Geometry: final body of the model. Coordinates: model frame, mm. Face numbers are marked on the shaded views. Round coordinates to 2 decimals unless told otherwise and drop trailing zeros. Loops run counter-clockwise (first coordinate to the right, second up) from the corner with the lowest first, then second, coordinate; pieces in that order, holes last. Notation, with made-up numbers: (2, 51) - (8, 51) arc R21 cw to (8, 66) - close; hole circle Ø6 at (43, -17). An arc over 180 degrees is marked (long way). Answer as a JSON object with one key per item and string values. Group by question number.
Item 1: Section B-B (y = 0). Return the cut outline in (x, z).
Item 2: Line query: line 1 (Y direction, x = 12, z = 0); line 2 (Z direction, x = 11.75, y = 3); line 3 (Y direction, x = 14, z = 6.5). Output: solid intervals per line, ascending.
Item 3: Section A-A (z = 0). Return the cut outline in (x, y), plus the area to 3 significant figures.
Item 4: Draft query along Y for the marked faces 1, 2 and 3. Return one class per face: released by +Y, released by -Y, zero draft, split by the parting line, or undercut.
Item 5: Section C-C (x = 6). Return the cut outline in (y, z).
```python
from build123d import *

# Parameters (mm, degrees)
SKETCH1_W           = 35
SKETCH1_H           = 30
BOSS_EXTRUDE1_DEPTH = 25
SKETCH2_R           = 8.23
CUT_EXTRUDE1_DEPTH  = 51
SKETCH3_W           = 35
SKETCH3_H           = 30
CUT_EXTRUDE2_DEPTH  = 5
SKETCH4_W           = 35
SKETCH4_H           = 30
CUT_EXTRUDE3_DEPTH  = 5


with BuildPart() as part:
    # Sketch1 → Boss-Extrude1 (new body)
    with BuildSketch(Plane(origin=(0, 0, 0), x_dir=(0, 0, -1), z_dir=(1, 0, 0))):
        Rectangle(SKETCH1_W, SKETCH1_H)
    extrude(amount=BOSS_EXTRUDE1_DEPTH)

    # Sketch2 → Cut-Extrude1 (cut)
    with BuildSketch(Plane(origin=(25, 0, 0), x_dir=(0, 0, -1), z_dir=(1, 0, 0))):
        Circle(SKETCH2_R)
    extrude(amount=-CUT_EXTRUDE1_DEPTH, mode=Mode.SUBTRACT)

    # Sketch3 → Cut-Extrude2 (cut)
    with BuildSketch(Plane(origin=(25, 0, 0), x_dir=(0, 0, -1), z_dir=(1, 0, 0))):
        Rectangle(SKETCH3_W, SKETCH3_H)
    extrude(amount=-CUT_EXTRUDE2_DEPTH, mode=Mode.SUBTRACT)

    # Sketch4 → Cut-Extrude3 (cut)
    with BuildSketch(Plane(origin=(20, 0, 0), x_dir=(0, 0, -1), z_dir=(1, 0, 0))):
        Rectangle(SKETCH4_W, SKETCH4_H)
    extrude(amount=-CUT_EXTRUDE3_DEPTH, mode=Mode.SUBTRACT)


solid = part.part
```
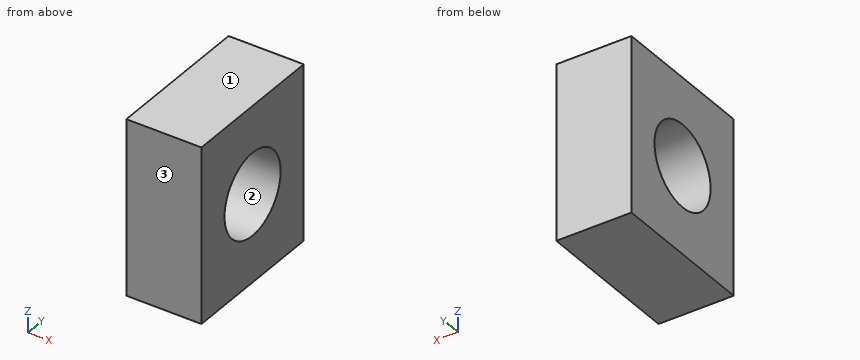
Values:
{
 "1": {"outline": "(0, -17.5) - (15, -17.5) - (15, -8.23) - (0, -8.23) - close; (0, 8.23) - (15, 8.23) - (15, 17.5) - (0, 17.5) - close"},
 "2": {"line 1": "y = -15 to -8.23, 8.23 to 15", "line 2": "z = -17.5 to -7.66, 7.66 to 17.5", "line 3": "y = -15 to -5.05, 5.05 to 15"},
 "3": {"outline": "(0, -15) - (15, -15) - (15, -8.23) - (0, -8.23) - close; (0, 8.23) - (15, 8.23) - (15, 15) - (0, 15) - close", "area": "203 mm^2"},
 "4": {"face 1": "zero draft", "face 2": "undercut", "face 3": "released by -Y"},
 "5": {"outline": "(-15, -17.5) - (15, -17.5) - (15, 17.5) - (-15, 17.5) - close; hole circle Ø16.46 at (0, 0)"}
}
